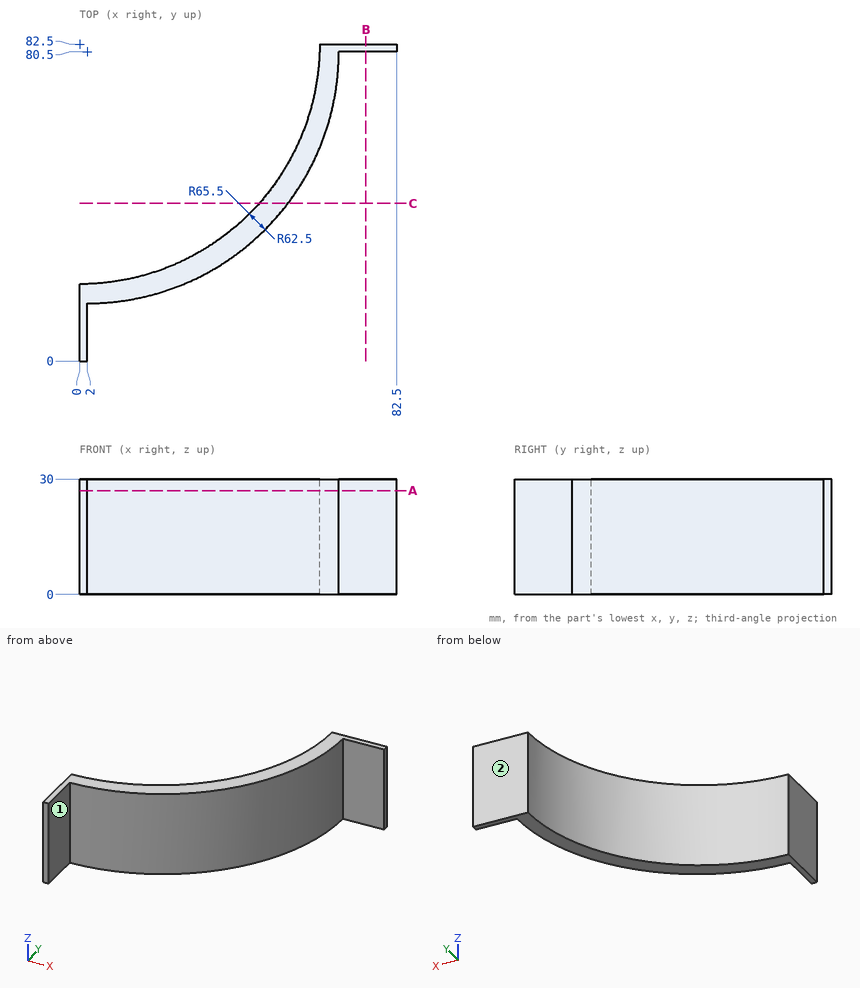
Design review of the part shown in the three views and the two pictorial views. Dimensions are in mm from the part's minimum x, y and z. A direction names the side the tool comes from. Coordinates: 2 decimals unless noted, no trailing zeros. Loops run counter-clockwise (first coordinate to the right, second up) from the corner with the lowest first, then second, coordinate; pieces in that order, holes last. Notation, with made-up numbers: (-13, 64) - (16, 64) arc R18 ccw to (16, 74) - close; hole circle Ø5 at (4.5, 73). An arc over 180 degrees is marked (long way). Use a Markdown table: item, result. Add a question column.
Item 1: We need section C-C (y = 41). Give the boundary of the cut face in (x, z).
Item 2: Tool access review of the marked faces 1 and 2: name each direction out of +Z, -Z, +X, -X, +Y, -Y from which nothing blocks a thin tool from reaching the whole face with its end or side.
Item 3: Insertion check: pin 1 Ø8 at (y, z) = (67, 23.5) entering from +X; pin 2 Ø6 at (y, z) = (18, 20) entering from -X; pin 3 Ø10 at (y, z) = (38, 14.5) entering from -X; pin 4 Ø8 at (x, z) = (40, 7.5) entering from -Y. Each pin has a flat end and moves straight along its axis. Give the tip position at first contact, or say it passes through.
Item 4: For line 1 (X direction, y = 11, z = 9.25); line 2 (Y direction, x = 75, z = 21.5); line 3 (Y direction, x = 47.5, z = 13.5), list the stretches that pass through material, from the lowest coordinate up.
Item 5: We need section A-A (z = 27). Give the boundary of the cut face in (x, y), and give its area (3 significant figures).
Item 6: We need section B-B (x = 74.5). Give the boundary of the cut face in (y, z), and give its area (3 significant figures).
Results list:
| question | item | result |
|---|---|---|
| 1 | outline | (46.73, 0) - (54.25, 0) - (54.25, 30) - (46.73, 30) - close |
| 2 | face 1 | +Z, -Z, +X, -Y |
| 2 | face 2 | +Z, -Z, +X, -X, +Y |
| 3 | pin 1 | stops at x = 66.81 |
| 3 | pin 2 | stops at x = 0 |
| 3 | pin 3 | stops at x = 38.16 |
| 3 | pin 4 | stops at y = 24.52 |
| 4 | line 1 | x = 0 to 2 |
| 4 | line 2 | y = 80.5 to 82.5 |
| 4 | line 3 | y = 33.38 to 41.88 |
| 5 | outline | (0, 0) - (2, 0) - (2, 15) arc R65.5 ccw to (67.5, 80.5) - (82.5, 80.5) - (82.5, 82.5) - (62.5, 82.5) arc R62.5 cw to (0, 20) - close |
| 5 | area | 628 mm^2 |
| 6 | outline | (80.5, 0) - (82.5, 0) - (82.5, 30) - (80.5, 30) - close |
| 6 | area | 60.0 mm^2 |
